from build123d import *

# Parameters (mm, degrees)
AUFSATZ_LINEAR_AUSTRAGEN1_DEPTH = 6.9
F_4_0_4_DURCHMESSER_BOHRUNG1_D  = 4
F_3_0_3_DURCHMESSER_BOHRUNG1_D  = 3


with BuildPart() as part:
    # Skizze1 → Aufsatz-Linear austragen1 (new body)
    with BuildSketch(Plane(origin=(0, 0, 0), x_dir=(1, 0, 0), z_dir=(0, 1, 0))):
        with BuildLine():
            Line((0, -3.95), (1, -3.95))
            ThreePointArc((1, -3.95), (2.530733729, -4.25448187), (3.828427125, -5.121572875))
            Line((3.828427125, -5.121572875), (7.131601718, -8.424747468))
            Line((7.131601718, -8.424747468), (21.273737342, 5.717388155))
            Line((21.273737342, 5.717388155), (5.717388155, 21.273737342))
            Line((5.717388155, 21.273737342), (-8.424747468, 7.131601718))
            Line((-8.424747468, 7.131601718), (-5.121572875, 3.828427125))
            ThreePointArc((-5.121572875, 3.828427125), (-4.25448187, 2.530733729), (-3.95, 1))
            Line((-3.95, 1), (-3.95, 0))
            ThreePointArc((-3.95, 0), (-2.793071786, -2.793071786), (0, -3.95))
        make_face()
    extrude(amount=AUFSATZ_LINEAR_AUSTRAGEN1_DEPTH)

    # Ø4.0 (4) Durchmesser Bohrung1 (through all)
    with Locations(Plane(origin=(0, 6.9, 0), x_dir=(1, 0, 0), z_dir=(0, 1, 0))):
        with Locations((-0.070710678, -0.070710678)):
            Hole(F_4_0_4_DURCHMESSER_BOHRUNG1_D / 2)

    # Ø3.0 (3) Durchmesser Bohrung1 (through all)
    with Locations(Plane(origin=(0, 6.9, 0), x_dir=(1, 0, 0), z_dir=(0, 1, 0))):
        with Locations((9.252922061, 9.252922061)):
            Hole(F_3_0_3_DURCHMESSER_BOHRUNG1_D / 2)


solid = part.part
Verification items for the finished model (mm, model axes). A direction names the side the tool comes from. Give positions to 0.01 mm unless a question says otherwise; leave off trailing zeros. Loops run counter-clockwise (first coordinate to the right, second up) from the corner with the lowest first, then second, coordinate; pieces in that order, holes last.
1. Cross-section at B-B on y = 4.75. Record the cut outline in (x, z), and give its area (3 significant figures).
Derived:
outline: (-8.42, -7.13) - (5.72, -21.27) - (21.27, -5.72) - (7.13, 8.42) - (3.83, 5.12) arc R4 cw to (1, 3.95) - (0, 3.95) arc R3.95 ccw to (-3.95, 0) - (-3.95, -1) arc R4 cw to (-5.12, -3.83) - close; hole circle Ø4 at (-0.07, 0.07); hole circle Ø3 at (9.25, -9.25)
area: 440 mm2
2. Tool access check on faces 4 (the flat face through (6, 6.9, -7)), 5 (the flat face through (0.5, 3.4, 3.95)). Record the directions out of +Z, -Z, +X, -X, +Y, -Y that give a thin tool (end or side, any length) a straight path to the whole face; none if there is none.
Derived:
face 4: +Z, -Z, +X, -X, +Y
face 5: +Z, -X, +Y, -Y
3. Go/stop test with flat-tipped pins: P1, Ø2, axis at x = 13, y = 3.5, coming from the +Z side; P2, Ø0.8, axis at x = 0.5, y = 3, coming from the +Z side; P3, Ø4, axis at x = 15.5, y = 4, coming from the -Z side. Record where each tip stops, or that it passes through.
Derived:
P1: stops at z = 3.56
P2: stops at z = 3.95
P3: stops at z = -13.49
4. Cross-section at A-A on z = -9.75. Record the cut outline in (x, y).
Derived:
outline: (-5.81, 0) - (7.84, 0) - (7.84, 6.9) - (-5.81, 6.9) - close; (10.67, 0) - (17.24, 0) - (17.24, 6.9) - (10.67, 6.9) - close
5. Cross-section at C-C on x = 1.5. Record the cut outline in (y, z), and give its area (3 significant figures).
Derived:
outline: (0, -17.06) - (6.9, -17.06) - (6.9, -1.17) - (0, -1.17) - close; (0, 1.31) - (6.9, 1.31) - (6.9, 3.98) - (0, 3.98) - close
area: 128 mm2
6. Material ranges on probe 1 along Z at (x, y) = (1, 1); probe 2 along X at (y, z) = (1, -8); probe 3 along X at (y, z) = (2.25, -9), recorded low to high.
Derived:
probe 1: z = -16.56 to -1.62, 1.76 to 3.95
probe 2: x = -7.56 to 8.43, 10.08 to 18.99
probe 3: x = -6.56 to 7.77, 10.73 to 17.99
7. Cross-section at D-D on x = 12.5. Record the cut outline in (y, z), and give its area (3 significant figures).
Derived:
outline: (0, -14.49) - (6.9, -14.49) - (6.9, 3.06) - (0, 3.06) - close
area: 121 mm2
8. Release check for a two-part mould opening along Z. For faces 1 (the cylindrical face through (0.19, 3.402, -1.912)), 2 (the flat face through (14.104, 3.402, 1.453)), 3 (the flat face through (-1.255, 3.402, -14.302)) record: +Z half, -Z half, draft (parallel to the pull), parting line (faces both ways), or undercut.
Derived:
face 1: undercut
face 2: +Z half
face 3: -Z half
